Autodesk Fusion 360 part; units mm, degrees
sketch "Sketch1" plane through (0, 0, 0) normal (0, 1, 0) x (1, 0, 0)
  line L0 (-12.15, 14.8) -> (-16.65, 14.8)
  line L1 (-16.65, 14.8) -> (-12.15, 14.8)
  line L2 (-12.15, 13.8) -> (-14.15, 13.8)
  line L3 (-15.15, -10.5) -> (-8, -10.5)
  line L4 (-8, -10.5) -> (-8, -12)
  line L5 (-8, -12) -> (-16.65, -12)
  line L6 (-12.15, 13.8) -> (-12.15, 14.8)
  line L7 (-14.15, 13.8) -> (-14.15, 11.5)
  line L8 (-14.15, 11.5) -> (-12.15, 11.5)
  line L9 (-12.15, 11.5) -> (-12.15, 10.5)
  line L10 (-12.15, 10.5) -> (-15.15, 10.5)
  line L11 (-16.65, 14.8) -> (-16.65, -12)
  line L12 (0, 6) -> (-15.15, 6)
  line L13 (-15.15, 6) -> (-15.15, 10.5)
  line L14 (0, 6) -> (0, 4.5)
  line L15 (0, 4.5) -> (-15.15, 4.5)
  line L16 (-15.15, 4.5) -> (-15.15, -10.5)
  dimension "d1" = 2.3
  dimension "d2" = 1
  dimension "d3" = 1
  dimension "d5" = 2
  dimension "d8" = 1.5
  dimension "d11" = 8
  dimension "d13" = 10.5
  dimension "d14" = 10.5
  dimension "d17" = 1
  dimension "d28" = 1.5
  dimension "d29" = 1.5
  dimension "d30" = 4.5
  dimension "d34" = 14.15
extrude "Extrude1" add sketch "Sketch1" along normal blind 5 makes body 1
chamfer "Chamfer1" distance 0.5 angle 45 3 edges at (-12.15, 2.5, -13.8) (-8, 2.5, 12) (-8, 2.5, 10.5) on bodies 1
fillet "Fillet1" radius 0.5 6 edges at (-8, 2.5, 11.5) (-8, 2.5, 11) (-8.5, 2.5, 12) (-8.5, 2.5, 10.5) (-12.15, 2.5, -14.3) (-12.65, 2.5, -13.8) on bodies 1
fillet "Fillet2" radius 2.3 4 edges at (-16.65, 2.5, 12) (-16.65, 2.5, -14.8) (-15.15, 2.5, -4.5) (-15.15, 2.5, 10.5) on bodies 1
fillet "Fillet3" radius 0.5 3 edges at (-12.15, 2.5, -14.8) (-12.15, 2.5, -11.5) (-12.15, 2.5, -10.5) on bodies 1
fillet "Fillet4" radius 1 2 edges at (-14.15, 2.5, -13.8) (-14.15, 2.5, -11.5) on bodies 1
fillet "Fillet5" radius 1.5 2 edges at (-15.15, 2.5, -10.5) (-15.15, 2.5, -6) on bodies 1
mirror "Mirror1" about plane through (0, 0, -6) normal (1, 0, 0) of bodies 1 makes body 2
combine "Combine1" operation add target body 1 tool bodies 2
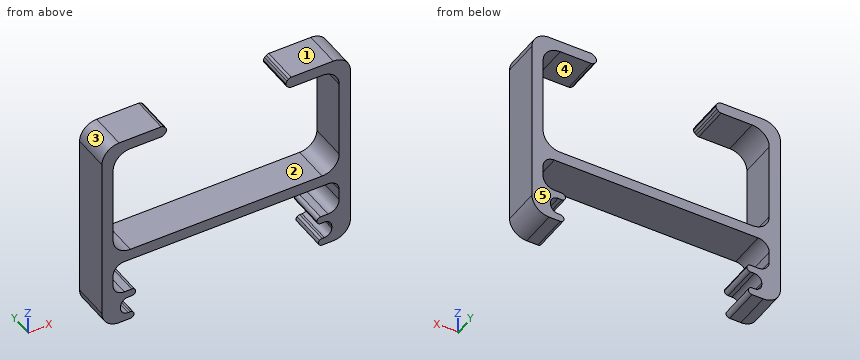
Check sheet for the modelled part. Datum: model origin and axes. Units: mm. Face numbers are marked on the shaded views. A direction names the side the tool comes from. Round coordinates to 2 decimals unless told otherwise and drop trailing zeros. Order: outer loops, then holes, each group sorted by start corner. A loop starts at its lowest first (then second) coordinate and runs counter-clockwise, first axis right, second up.
1) Scan lines: line 1 (Z direction, x = -13, y = 4.1); line 2 (X direction, y = 3.05, z = 2.25); line 3 (Z direction, x = 0, y = 2.45). Record each from-to range of solid material in increasing order.
2) Go/stop test with flat-tipped pins: pin 1 Ø1.2 at (x, y) = (-11, 3.5) entering from -Z; pin 2 Ø1 at (x, y) = (-2.5, 3) entering from +Z. Record where each tip stops, or that it passes through.
3) Section check B-B (z = -6.75). Record the boundary of the cut face in (x, y).
4) Mould release check, pull along X, two halves, no side actions. Record for the marked faces 3, 4 and 5: +X half, -X half, draft (parallel to the pull), parting line (faces both ways), or undercut.
5) Tool access check on the marked faces 1 and 2. Record the directions out of +Z, -Z, +X, -X, +Y, -Y that give a thin tool (end or side, any length) a straight path to the whole face; none if there is none.
6) Section check C-C (x = -0.5). Record the boundary of the cut face in (y, z), and give its area (3 significant figures).
7) Section check A-A (z = -1.5). Record the boundary of the cut face in (x, y), and give its area (3 significant figures).
Result:
1. line 1: z = -14.8 to -13.8, -11.5 to -10.5, -6 to -4.5, 10.5 to 12
1. line 2: x = -16.65 to -15.15, 15.15 to 16.65
1. line 3: z = -6 to -4.5
2. pin 1: stops at z = -6
2. pin 2: stops at z = -4.5
3. outline: (-16.65, 0) - (-14.95, 0) - (-14.95, 5) - (-16.65, 5) - close; (14.95, 0) - (16.65, 0) - (16.65, 5) - (14.95, 5) - close
4. face 3: -X half
4. face 4: undercut
4. face 5: draft
5. face 1: +Z, +X, -X, +Y, -Y
5. face 2: +Y, -Y
6. outline: (0, -6) - (5, -6) - (5, -4.5) - (0, -4.5) - close
6. area: 7.50 mm2
7. outline: (-16.65, 0) - (-15.15, 0) - (-15.15, 5) - (-16.65, 5) - close; (15.15, 0) - (16.65, 0) - (16.65, 5) - (15.15, 5) - close
7. area: 15.0 mm2
